```python
from build123d import *

# Parameters (mm, degrees)
BOSS_EXTRUDE1_DEPTH = 3.2
BOSS_EXTRUDE2_DEPTH = 1.8
BOSS_EXTRUDE3_DEPTH = 3.2


with BuildPart() as part:
    # Sketch1 → Boss-Extrude1 (new body)
    with BuildSketch(Plane.XY):
        with BuildLine():
            Line((-3, 4.582902076), (-3, 0))
            Line((-3, 0), (0, 0))
            Line((0, 0), (0, 5))
            Line((0, 5), (-1.00094518, 5))
            ThreePointArc((-1.00094518, 5), (-2.021997437, 4.894614703), (-3, 4.582902076))
        make_face()
    extrude(amount=BOSS_EXTRUDE1_DEPTH)

    # Sketch2 → Boss-Extrude2 (add)
    with BuildSketch(Plane(origin=(0, 0, 0), x_dir=(-1, 0, 0), z_dir=(0, 0, -1))):
        with BuildLine():
            Line((3, 0), (5.973192614, 0))
            ThreePointArc((5.973192614, 0), (5.167805035, 2.733390386), (3, 4.582902076))
            Line((3, 4.582902076), (3, 0))
        make_face()
    extrude(amount=-BOSS_EXTRUDE2_DEPTH)

    # Sketch3 → Boss-Extrude3 (add)
    with BuildSketch(Plane.XY.offset(1.8)):
        with BuildLine():
            Line((0, 0), (-5.973207287, 0.012113161))
            add(Edge.make_bspline(
                [(-5.973207287, 0.012113161), (-2.989270297, 3.993959552), (0, 0)],
                knots=[0, 0, 0, 1, 1, 1], degree=2))
        make_face()
    extrude(amount=BOSS_EXTRUDE3_DEPTH)


solid = part.part
```
Source: CAD feature listing. Evaluate the final solid. Frame: model axes, mm. A direction names the side the tool comes from. Coordinates: 2 decimals unless noted, no trailing zeros. Write each loop counter-clockwise with the first axis right and the second up, starting at its lowest first coordinate (ties: lowest second). Pieces come first, ordered by that corner, then holes. Notation, with made-up numbers: (18.25, 85.5) -> (56.25, 85.5) arc R12 cw to (56.25, 90.5) -> close; hole circle Ø9 at (47, 45.25). An arc over 180 degrees is marked (long way). Return JSON: item names as keys, results as strings. Group by question number.
1) Section query A-A, the plane z = 1.6. Return loops of the section in (x, y).
2) Ray query, line 1 along Z through (x, y) = (-1.35, 2.6); line 2 along Z through (x, y) = (-5.2, 1.8); line 3 along X through (y, z) = (3.7, 2.6). Return the intervals inside material, ascending.
3) Set-up query: faces 1 (the face through (-4, 2, 1.8)), 2 (the face through (-2, 0, 1)), 3 (the face through (-2, 3, 3.2)). Return all of +Z, -Z, +X, -X, +Y, -Y with unobstructed straight access to the full face (end or side cutting, diameter ignored); none if empty.
4) Contact query for a flat-ended pin moving along its axis: P1, Ø3, axis at x = -5, z = 1, coming from the +Y side. Output: stop coordinate, or through.
5) Section query B-B, the plane y = 3.3. Return loops of the section in (x, z), plus the area to 3 significant figures.
6) Section query C-C, the plane y = 2.75. Return loops of the section in (x, z), plus the area to 3 significant figures.
From the geometry:
{
 "1": {"outline": "(-5.97, 0) -> (0, 0) -> (0, 5) -> (-1, 5) arc R5 ccw to (-3, 4.58) arc R5 ccw to start"},
 "2": {"line 1": "0 to 3.2", "line 2": "0 to 1.8", "line 3": "-3 to 0"},
 "3": {"face 1": "+Z, -X, +Y", "face 2": "+Z, -Z, +X, -X, -Y", "face 3": "+Z, +X, +Y"},
 "4": {"P1": "y = 4.33"},
 "5": {"outline": "(-4.74, 0) -> (0, 0) -> (0, 3.2) -> (-3, 3.2) -> (-3, 1.8) -> (-4.74, 1.8) -> close", "area": "12.7 mm²"},
 "6": {"outline": "(-5.16, 0) -> (0, 0) -> (0, 3.2) -> (-3, 3.2) -> (-3, 1.8) -> (-5.16, 1.8) -> close", "area": "13.5 mm²"}
}
